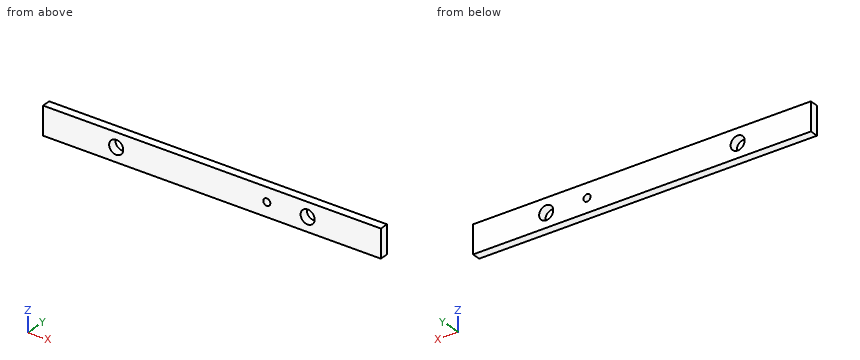
```python
from build123d import *

# Parameters (mm, degrees)
SKETCH3_W           = 120
SKETCH3_H           = 10
BOSS_EXTRUDE1_DEPTH = 3
SKETCH5_R           = 2.5
SKETCH5_R_2         = 1.25
CUT_EXTRUDE1_DEPTH  = 3


with BuildPart() as part:
    # Sketch3 → Boss-Extrude1 (new body)
    with BuildSketch(Plane(origin=(0, 0, 0), x_dir=(1, 0, 0), z_dir=(0, 1, 0))):
        Rectangle(SKETCH3_W, SKETCH3_H)
    extrude(amount=BOSS_EXTRUDE1_DEPTH)

    # Sketch5 → Cut-Extrude1 (cut)
    with BuildSketch(Plane(origin=(0, 0, 0), x_dir=(1, 0, 0), z_dir=(0, 1, 0))):
        with Locations(Location((-34, 0, 0), (0, 0, 90))):
            Circle(SKETCH5_R)
        with Locations(Location((34, 0, 0), (0, 0, 90))):
            Circle(SKETCH5_R)
        with Locations(Location((19.5, 0, 0), (0, 0, 90))):
            Circle(SKETCH5_R_2)
    extrude(amount=CUT_EXTRUDE1_DEPTH, mode=Mode.SUBTRACT)


solid = part.part
```
The model under review builds one solid part; all positions refer to its coordinate system, in mm. Round coordinates to 2 decimals unless told otherwise and drop trailing zeros. Loops run counter-clockwise (first coordinate to the right, second up) from the corner with the lowest first, then second, coordinate; pieces in that order, holes last. Notation, with made-up numbers: (2.25, 70) - (30.25, 70) arc R30 cw to (30.25, 99) - close; hole circle Ø6 at (81, -23). An arc over 180 degrees is marked (long way). Use a Markdown table: item, result. Add a question column.
Q1. Add section A-A (z = 0). State the section outline as (x, y) points.
Q2. Add section D-D (x = 19.5). State the section outline as (y, z) points, plus the area to 3 significant figures.
Q3. For probe 1 along X at (y, z) = (1.6, 0); probe 2 along Z at (x, y) = (34, 1.1); probe 3 along Z at (x, y) = (19.5, 2.45), list the stretches that pass through material, from the lowest coordinate up.
Q4. Insertion check: pin 1 Ø4.5 at (x, z) = (-34, 0) entering from -Y. The pin has a flat end and moves straight along its axis. Give the tip position at first contact, or say it passes through.
Q5. Add section C-C (y = 1.05). State the section outline as (x, z) points, plus the area to 3 significant figures.
Q6. Add section B-B (x = 34). State the section outline as (y, z) points.
Worked answers:
| question | item | result |
|---|---|---|
| 1 | outline | (-60, 0) - (-36.5, 0) - (-36.5, 3) - (-60, 3) - close; (-31.5, 0) - (18.25, 0) - (18.25, 3) - (-31.5, 3) - close; (20.75, 0) - (31.5, 0) - (31.5, 3) - (20.75, 3) - close; (36.5, 0) - (60, 0) - (60, 3) - (36.5, 3) - close |
| 2 | outline | (0, -5) - (3, -5) - (3, -1.25) - (0, -1.25) - close; (0, 1.25) - (3, 1.25) - (3, 5) - (0, 5) - close |
| 2 | area | 22.5 mm² |
| 3 | probe 1 | -60 to -36.5, -31.5 to 18.25, 20.75 to 31.5, 36.5 to 60 |
| 3 | probe 2 | -5 to -2.5, 2.5 to 5 |
| 3 | probe 3 | -5 to -1.25, 1.25 to 5 |
| 4 | pin 1 | through |
| 5 | outline | (-60, -5) - (60, -5) - (60, 5) - (-60, 5) - close; hole circle Ø5 at (-34, 0); hole circle Ø2.5 at (19.5, 0); hole circle Ø5 at (34, 0) |
| 5 | area | 1,160 mm² |
| 6 | outline | (0, -5) - (3, -5) - (3, -2.5) - (0, -2.5) - close; (0, 2.5) - (3, 2.5) - (3, 5) - (0, 5) - close |
